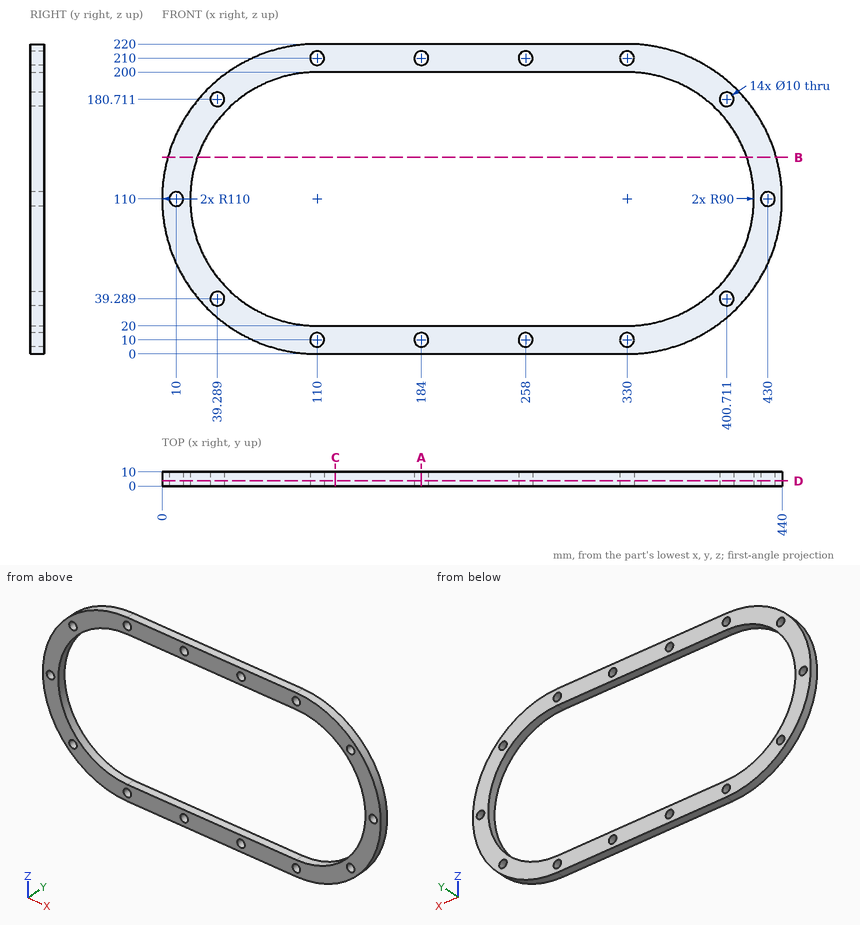
Verification items for this drawing (mm, ordinates from the low corner). Coordinates: 2 decimals unless noted, no trailing zeros. Loops run counter-clockwise (first coordinate to the right, second up) from the corner with the lowest first, then second, coordinate; pieces in that order, holes last. Notation, with made-up numbers: (29, 19.5) -> (46, 19.5) arc R6 ccw to (46, 28.5) -> close; hole circle Ø5 at (10, 68). An arc over 180 degrees is marked (long way). Answer in a Markdown table with one row per item. Add a question column.
1. Section check B-B, the plane z = 139.5. Enter the section's corners in (x, y).
2. Material ranges on probe 1 along Z at (x, y) = (330, 6); probe 2 along Z at (x, y) = (311, 7.5); probe 3 along Z at (x, y) = (183, 4.5), recorded low to high. Write a range as [from, to].
3. Depth check by flat-ended pin: P1, Ø1.5, axis at y = 6, z = 131, coming from the +X side; P2, Ø6, axis at x = 80.5, y = 6.5, coming from the -Z side; P3, Ø8, axis at x = 39.29, z = 39.29, coming from the +Y side. Enter the tip coordinate at first touch or a pass-through.
4. Section check D-D, the plane y = 3.75. Give the number of separate pieces and of enclosed holes in the cut face, then the cut area to 3 significant figures.
5. Section check C-C, the plane x = 123. Enter the section's corners in (y, z).
6. Section check A-A, the plane x = 184. Enter the section's corners in (y, z), then the cut area to 3 significant figures.
Derived:
| question | item | result |
|---|---|---|
| 1 | outline | (4.03, 0) -> (24.97, 0) -> (24.97, 10) -> (4.03, 10) -> close; (415.03, 0) -> (435.97, 0) -> (435.97, 10) -> (415.03, 10) -> close |
| 2 | probe 1 | z = [0, 5], [15, 20], [200, 205], [215, 220] |
| 2 | probe 2 | z = [0, 20], [200, 220] |
| 2 | probe 3 | z = [0, 5.1], [14.9, 20], [200, 205.1], [214.9, 220] |
| 3 | P1 | stops at x = 438.12 |
| 3 | P2 | stops at z = 3.24 |
| 3 | P3 | passes through |
| 4 | separate pieces | 1 |
| 4 | enclosed holes | 15 |
| 4 | area | 20,300 mm² |
| 5 | outline | (0, 0) -> (10, 0) -> (10, 20) -> (0, 20) -> close; (0, 200) -> (10, 200) -> (10, 220) -> (0, 220) -> close |
| 6 | outline | (0, 0) -> (10, 0) -> (10, 5) -> (0, 5) -> close; (0, 15) -> (10, 15) -> (10, 20) -> (0, 20) -> close; (0, 200) -> (10, 200) -> (10, 205) -> (0, 205) -> close; (0, 215) -> (10, 215) -> (10, 220) -> (0, 220) -> close |
| 6 | area | 200 mm² |
